from build123d import *

# Parameters (mm, degrees)
SKETCH1_W           = 108.320866354
SKETCH1_H           = 20
SKETCH1_R           = 1.5
SKETCH1_W_2         = 96.320866354
SKETCH1_H_2         = 12
BOSS_EXTRUDE1_DEPTH = 6
CUT_EXTRUDE1_DEPTH  = 111.315049234
FILLET1_R           = 5


with BuildPart() as part:
    # Sketch1 → Boss-Extrude1 (new body)
    with BuildSketch(Plane(origin=(0, 0, 0), x_dir=(1, 0, 0), z_dir=(0, 1, 0))):
        with Locations((54.160433177, 10)):
            Rectangle(SKETCH1_W, SKETCH1_H)
        with Locations(Location((3, 17, 0), (0, 0, 270))):
            Circle(SKETCH1_R, mode=Mode.SUBTRACT)
        with Locations(Location((3, 3, 0), (0, 0, 90))):
            Circle(SKETCH1_R, mode=Mode.SUBTRACT)
        with Locations(Location((105.320866354, 3, 0), (0, 0, 270))):
            Circle(SKETCH1_R, mode=Mode.SUBTRACT)
        with Locations(Location((105.320866354, 17, 0), (0, 0, 90))):
            Circle(SKETCH1_R, mode=Mode.SUBTRACT)
        with Locations((54.160433177, 10)):
            Rectangle(SKETCH1_W_2, SKETCH1_H_2, mode=Mode.SUBTRACT)
    extrude(amount=BOSS_EXTRUDE1_DEPTH)

    # Sketch2 → Cut-Extrude1 (cut, through all)
    with BuildSketch(Plane(origin=(0, 6, 0), x_dir=(1, 0, 0), z_dir=(0, 1, 0))):
        Polygon((89.320866354, 17), (89.320866354, 16), (102.320866354, 16), (102.320866354, 4), (89.320866354, 4), (89.320866354, 3), (103.320866354, 3), (103.320866354, 17), align=None)
    extrude(amount=-CUT_EXTRUDE1_DEPTH, mode=Mode.SUBTRACT)

    # Fillet1
    # the kernel refuses this fillet: 5 mm, written as the material it adds along each edge
    with BuildSketch(Plane(origin=(103.320866354, 6, -17), x_dir=(0, 0, 1), z_dir=(0, -1, 0)), Plane(origin=(103.320866354, 6, -3), x_dir=(-1, 0, 0), z_dir=(0, -1, 0)), Plane(origin=(6, 0, -16), x_dir=(0, 0, 1), z_dir=(0, 1, 0))) as fillet1_piece_1:
        with BuildLine():
            CenterArc((FILLET1_R, FILLET1_R), FILLET1_R, 180, 90)
            Line((0, FILLET1_R), (-FILLET1_R * 0.02, FILLET1_R))
            Line((-FILLET1_R * 0.02, FILLET1_R), (-FILLET1_R * 0.02, -FILLET1_R * 0.02))
            Line((-FILLET1_R * 0.02, -FILLET1_R * 0.02), (FILLET1_R, -FILLET1_R * 0.02))
            Line((FILLET1_R, -FILLET1_R * 0.02), (FILLET1_R, 0))
        make_face()
    extrude(amount=6)
    with BuildSketch(Plane(origin=(89.320866354, 6, -17), x_dir=(1, 0, 0), z_dir=(0, -1, 0))) as fillet1_piece_2:
        with BuildLine():
            CenterArc((3, 5), FILLET1_R, 233.130102354, 36.869897646)
            Line((0, 1), (-0.06, 0.92))
            ThreePointArc((-0.06, 0.92), (-0.1, 0.5), (-0.1, 0))
            Line((-0.1, 0), (0, -0.1))
            Line((0, -0.1), (3, -0.1))
            Line((3, -0.1), (3, 0))
        make_face()
    extrude(amount=6)
    with BuildSketch(Plane(origin=(89.320866354, 6, -3), x_dir=(0, 0, -1), z_dir=(0, -1, 0))) as fillet1_piece_3:
        with BuildLine():
            CenterArc((5, 3), FILLET1_R, 180, 36.869897646)
            Line((0, 3), (-0.1, 3))
            Line((-0.1, 3), (-0.1, 0))
            Line((-0.1, 0), (0, -0.1))
            ThreePointArc((0, -0.1), (0.5, -0.1), (0.92, -0.06))
            Line((0.92, -0.06), (1, 0))
        make_face()
    extrude(amount=6)
    with BuildSketch(Plane(origin=(6, 0, -4), x_dir=(0, 0, -1), z_dir=(0, 1, 0))) as fillet1_piece_4:
        with BuildLine():
            CenterArc((FILLET1_R, -FILLET1_R), FILLET1_R, 90, 90)
            Line((0, -FILLET1_R), (-FILLET1_R * 0.02, -FILLET1_R))
            Line((-FILLET1_R * 0.02, -FILLET1_R), (-FILLET1_R * 0.02, FILLET1_R * 0.02))
            Line((-FILLET1_R * 0.02, FILLET1_R * 0.02), (FILLET1_R, FILLET1_R * 0.02))
            Line((FILLET1_R, FILLET1_R * 0.02), (FILLET1_R, 0))
        make_face()
    extrude(amount=6)


solid = part.part
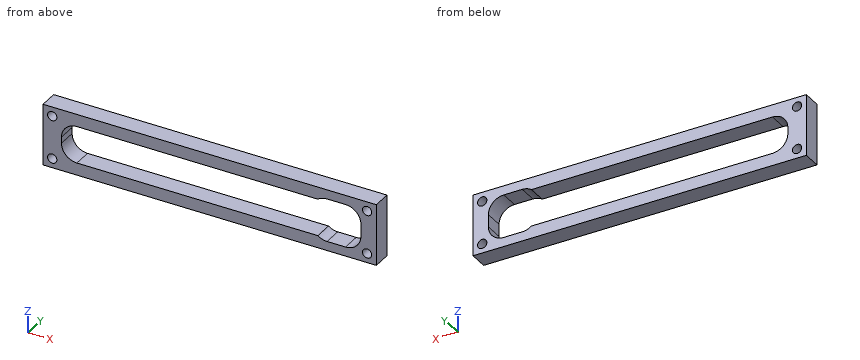
The listing builds one solid part. Answer for the finished solid, in the listing's coordinates (mm). Round coordinates to 2 decimals unless told otherwise and drop trailing zeros. Write each loop counter-clockwise with the first axis right and the second up, starting at its lowest first coordinate (ties: lowest second). Pieces come first, ordered by that corner, then holes. Notation, with made-up numbers: M 83.25,42.25 L 92.25,42.25 A24 ccw 92.25,70.25 Z; hole C 65.5,79.5 d7. An arc over 180 degrees is marked long. Write each question's results on one line, items separated by ' | '. Start each with the question number.
Item 1: A cutting plane is placed at C-C on z = -14. Write down the section's boundary in (x, y).
Item 2: A cutting plane is placed at A-A on x = 3. Write down the section's boundary in (y, z).
Item 3: A cutting plane is placed at D-D on y = 4.7. Write down the section's boundary in (x, z), and give its area (3 significant figures).
Item 4: Straight lines are drawn through the part: L1, parallel to Z at x = 11, y = 1.95; L2, parallel to Z at x = 96.5, y = 5.4; L3, parallel to X at y = 1.75, z = -11.25. For each, find the intervals that lie inside material, in ascending order. Write a range as [from, to].
Item 5: A flat-ended cylindrical pin translates along its axis: pin 1 Ø2.5 at (x, z) = (3, -17) entering from +Y. Find the tip coordinate at first contact, or state that the pin passes through.
Item 6: A cutting plane is placed at B-B on x = 97. Write down the section's boundary in (y, z), and give its area (3 significant figures).
Check sheet entries:
1) outline: M 0,0 L 7,0 L 7,6 L 0,6 Z; M 102.9,0 L 108.32,0 L 108.32,6 L 102.9,6 Z
2) outline: M 0,-20 L 6,-20 L 6,-18.5 L 0,-18.5 Z; M 0,-15.5 L 6,-15.5 L 6,-4.5 L 0,-4.5 Z; M 0,-1.5 L 6,-1.5 L 6,0 L 0,0 Z
3) outline: M 0,-20 L 108.32,-20 L 108.32,0 L 0,0 Z; hole C 3,-17 d3; hole C 3,-3 d3; hole M 6,-11 A5 ccw 11,-16 L 89.32,-16 A5 ccw 92.32,-17 L 98.32,-17 A5 ccw 103.32,-12 L 103.32,-8 A5 ccw 98.32,-3 L 92.32,-3 A5 ccw 89.32,-4 L 11,-4 A5 ccw 6,-9 Z; hole C 105.32,-17 d3; hole C 105.32,-3 d3 | area: 966 mm²
4) L1: [-20, -16], [-4, 0] | L2: [-20, -17], [-3, 0] | L3: [0, 6.01], [103.32, 108.32]
5) pin 1: through
6) outline: M 0,-20 L 6,-20 L 6,-17 L 0,-17 Z; M 0,-3 L 6,-3 L 6,0 L 0,0 Z | area: 36.0 mm²
